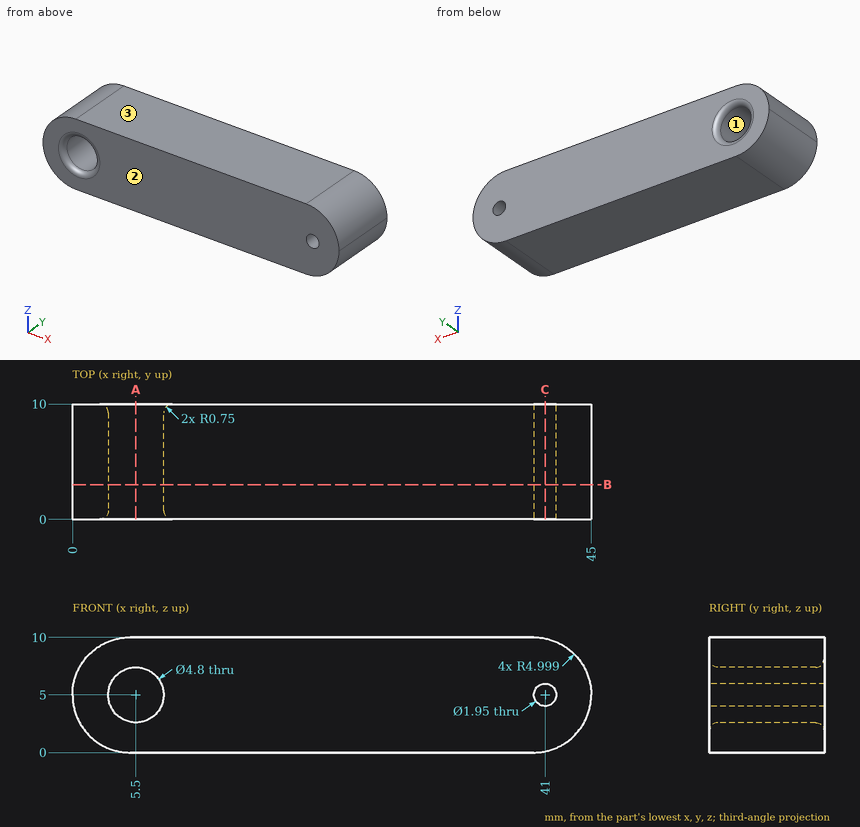
Answer from the drawing. Dimensions are ordinates in mm from the lowest x, y and z of the part. Coordinates: 2 decimals unless noted, no trailing zeros. Loops run counter-clockwise (first coordinate to the right, second up) from the corner with the lowest first, then second, coordinate; pieces in that order, holes last.
1) Section B-B (y = 3) is taken. Give the number of separate pieces and of enclosed holes in the cut face, plus the area to 3 significant figures.
Results:
separate pieces: 1
enclosed holes: 2
area: 407 mm2
2) For a pull along Z with two mould halves and no side action, classify the marked faces 1, 2 and 3 as +Z half, -Z half, draft (parallel to the pull), parting line (faces both ways), or undercut.
Results:
face 1: undercut
face 2: draft
face 3: +Z half
3) Flat-ended cylindrical pins translate along their axes: pin 1 (6 mm diameter, centred on y = 9, z = 9, fed in from +X); pin 2 (1 mm diameter, centred on y = 3.5, z = 2, fed in from -X). Find the tip coordinate at first contact, or state that the pin passes through.
Results:
pin 1: stops at x = 44.9
pin 2: stops at x = 0.67
4) Consider probe 1 along X at (y, z) = (2.75, 5) (3 decimals); probe 2 along Z at (x, y) = (5.5, 2.5); probe 3 along X at (y, z) = (5.5, 5.75). Determine where each line is inside the solid, lowest interval first.
Results:
probe 1: x = 0 to 3.1, 7.9 to 40.025, 41.975 to 45
probe 2: z = 0 to 2.6, 7.4 to 10
probe 3: x = 0.06 to 3.22, 7.78 to 40.38, 41.62 to 44.94
5) Section A-A (x = 5.5) is taken. Give the vertices of the cut face in (y, z), plus the area to 3 significant figures.
Results:
outline: (0, 0) - (10, 0) - (10, 1.85) arc R0.75 ccw to (9.25, 2.6) - (0.75, 2.6) arc R0.75 ccw to (0, 1.85) - close; (0, 8.15) arc R0.75 ccw to (0.75, 7.4) - (9.25, 7.4) arc R0.75 ccw to (10, 8.15) - (10, 10) - (0, 10) - close
area: 51.5 mm2
6) Section C-C (x = 41) is taken. Give the vertices of the cut face in (y, z) (3 decimals), plus the area to 3 significant figures.
Results:
outline: (0, 0.101) - (10, 0.101) - (10, 4.025) - (0, 4.025) - close; (0, 5.975) - (10, 5.975) - (10, 9.899) - (0, 9.899) - close
area: 78.5 mm2
